from build123d import *

# Parameters (mm, degrees)
SKETCH1_W                = 35
SKETCH1_H                = 18
BOSS_EXTRUDE1_DEPTH      = 8
SKETCH2_W                = 3
SKETCH2_H                = 6.1
CUT_EXTRUDE1_DEPTH       = 36
SKETCH3_W                = 3
SKETCH3_H                = 6.1
CUT_EXTRUDE2_DEPTH       = 36
M2_CLEARANCE_HOLE1_D     = 2.459
M2_CLEARANCE_HOLE1_DEPTH = 8
CHAMFER1_SIZE            = 0.2705
CHAMFER2_SIZE            = 2
SKETCH6_W                = 35
SKETCH6_H                = 1
CUT_EXTRUDE4_DEPTH       = 10


with BuildPart() as part:
    # Sketch1 → Boss-Extrude1 (new body)
    with BuildSketch(Plane.XY.offset(8)):
        Rectangle(SKETCH1_W, SKETCH1_H)
    extrude(amount=-BOSS_EXTRUDE1_DEPTH)

    # Sketch2 → Cut-Extrude1 (cut, through all)
    with BuildSketch(Plane.ZY.offset(17.5)):
        with Locations((6.5, 5.95)):
            Rectangle(SKETCH2_W, SKETCH2_H)
    extrude(amount=-CUT_EXTRUDE1_DEPTH, mode=Mode.SUBTRACT)

    # Sketch3 → Cut-Extrude2 (cut, through all)
    with BuildSketch(Plane.ZY.offset(17.5)):
        with Locations((6.5, -5.95)):
            Rectangle(SKETCH3_W, SKETCH3_H)
    extrude(amount=-CUT_EXTRUDE2_DEPTH, mode=Mode.SUBTRACT)

    # M2 Clearance Hole1
    with Locations(Plane.XY.offset(8)):
        with Locations((-10, 0), (10, 0)):
            Hole(M2_CLEARANCE_HOLE1_D / 2, depth=M2_CLEARANCE_HOLE1_DEPTH)

    # Chamfer1
    chamfer1_edges = [part.edges().sort_by_distance(p)[0] for p in [
        (11.2295, 0, 8),
        (11.2295, 0, 0),
        (-8.7705, 0, 8),
        (-8.7705, 0, 0),
    ]]
    chamfer(chamfer1_edges, length=CHAMFER1_SIZE)

    # Chamfer2
    chamfer2_edges = [part.edges().sort_by_distance(p)[0] for p in [
        (17.5, 5.95, 5),
        (17.5, 2.9, 6.5),
        (-17.5, 5.95, 5),
        (-17.5, 2.9, 6.5),
        (17.5, -5.95, 5),
        (17.5, -2.9, 6.5),
        (-17.5, -2.9, 6.5),
        (-17.5, -5.95, 5),
    ]]
    chamfer(chamfer2_edges, length=CHAMFER2_SIZE)

    # Sketch6 → Cut-Extrude4 (cut)
    with BuildSketch(Plane(origin=(0, 2.9, 0), x_dir=(1, 0, 0), z_dir=(0, 1, 0))):
        with Locations((0, -7.5)):
            Rectangle(SKETCH6_W, SKETCH6_H)
    extrude(amount=-CUT_EXTRUDE4_DEPTH, mode=Mode.SUBTRACT)


solid = part.part
Check sheet for the modelled part. Datum: model origin and axes. Units: mm. A direction names the side the tool comes from. Round coordinates to 2 decimals unless told otherwise and drop trailing zeros. Loops run counter-clockwise (first coordinate to the right, second up) from the corner with the lowest first, then second, coordinate; pieces in that order, holes last. Notation, with made-up numbers: (-10, -1) -> (23, -1) arc R31 ccw to (23, 31) -> close; hole circle Ø10 at (-14.5, 27). An arc over 180 degrees is marked (long way). Put each result on its own line as item: value. Start each with the question number.
1. Section check A-A (z = 4.25). Enter the section's corners in (x, y), plus the area to 3 significant figures.
2. Scan lines: probe 1 along Y at (x, z) = (-10, 1.75); probe 2 along X at (y, z) = (1, 1); probe 3 along Z at (x, y) = (-12.5, -4). Record each from-to range of solid material in increasing order.
3. Draft check along X on faces 6 (the face through (-16.5, -5.9, 4)), 7 (the face through (0, -2.9, 6)), 8 (the face through (-11.173, 0.369, 3.588)), 9 (the face through (16.5, 5.9, 4)). Enter one of: +X half, -X half, draft (parallel to the pull), parting line (faces both ways), or undercut.
4. Section check B-B (y = -2.25). Enter the section's corners in (x, z).
5. Section check C-C (x = -10). Enter the section's corners in (y, z).
6. Access from +Z, -Z, +X, -X, +Y, -Y to the whole of each face (thin tool, end or side, straight path). Record for faces 1 (the face through (0, -6, 5)), 2 (the face through (-16.5, -1.9, 5.4)), 3 (the face through (-16.5, 5.8, 4)), 4 (the face through (16.5, -1.9, 5.5)), 5 (the face through (0, 2.9, 6)).
7. Gauge pin test, flat ends, axial feed: pin 1 (3 mm diameter, centred on x = -9.5, y = 5.5, fed in from +Z); pin 2 (2 mm diameter, centred on x = 0, z = 6.5, fed in from -Y). Record the tip position at first contact, or that the pin passes through.
8. Section check D-D (y = 0). Enter the section's corners in (x, z).
Findings:
1. outline: (-17.5, -0.9) -> (-16.25, -2.15) -> (-16.25, -9) -> (16.25, -9) -> (16.25, -2.15) -> (17.5, -0.9) -> (17.5, 0.9) -> (16.25, 2.15) -> (16.25, 9) -> (-16.25, 9) -> (-16.25, 2.15) -> (-17.5, 0.9) -> close; hole circle Ø2.46 at (-10, 0); hole circle Ø2.46 at (10, 0)
1. area: 583 mm^2
2. probe 1: y = -9 to -1.23, 1.23 to 9
2. probe 2: x = -17.5 to -10.72, -9.28 to 9.28, 10.72 to 17.5
2. probe 3: z = 0 to 5
3. face 6: -X half
3. face 7: draft
3. face 8: undercut
3. face 9: +X half
4. outline: (-17.5, 0) -> (17.5, 0) -> (17.5, 3) -> (16.15, 4.35) -> (16.15, 7) -> (-16.15, 7) -> (-16.15, 4.35) -> (-17.5, 3) -> close
5. outline: (-9, 0) -> (-1.5, 0) -> (-1.23, 0.27) -> (-1.23, 7) -> (-2.9, 7) -> (-2.9, 5) -> (-9, 5) -> close; (1.23, 0.27) -> (1.5, 0) -> (9, 0) -> (9, 5) -> (2.9, 5) -> (2.9, 7) -> (1.23, 7) -> close
6. face 1: +Z, +X, -X, -Y
6. face 2: +Z, -X, -Y
6. face 3: +Z, -X, +Y
6. face 4: +Z, +X, -Y
6. face 5: +Z, +X, -X, +Y
7. pin 1: stops at z = 5
7. pin 2: stops at y = -2.9
8. outline: (-17.5, 0) -> (-11.5, 0) -> (-11.23, 0.27) -> (-11.23, 7) -> (-17.5, 7) -> close; (-8.77, 0.27) -> (-8.5, 0) -> (8.5, 0) -> (8.77, 0.27) -> (8.77, 7) -> (-8.77, 7) -> close; (11.23, 0.27) -> (11.5, 0) -> (17.5, 0) -> (17.5, 7) -> (11.23, 7) -> close
